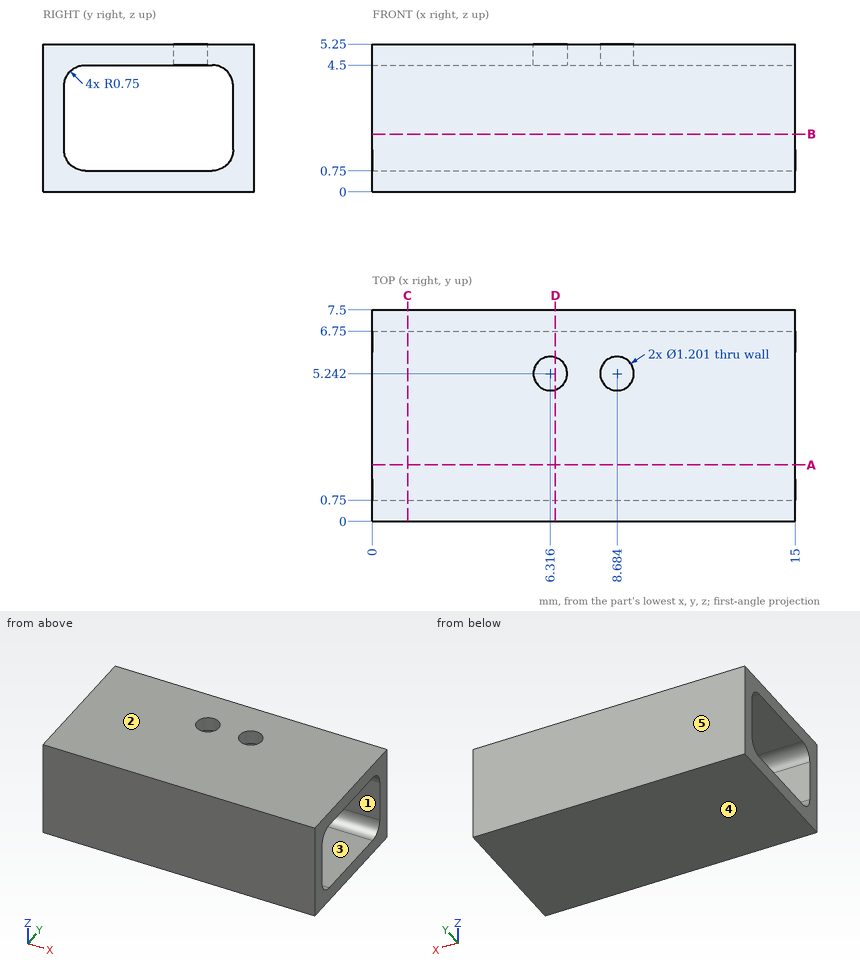
Verification items for this drawing (mm, ordinates from the low corner). A direction names the side the tool comes from. Round coordinates to 2 decimals unless told otherwise and drop trailing zeros. Loops run counter-clockwise (first coordinate to the right, second up) from the corner with the lowest first, then second, coordinate; pieces in that order, holes last. Notation, with made-up numbers: (43.25, 66.25) - (73.25, 66.25) arc R16 cw to (73.25, 82.25) - close; hole circle Ø9 at (68, -40). An arc over 180 degrees is marked (long way). Answer as CSV lines item,"result". Start each with the question number.
Item 1: Set-up check for the marked faces 1 and 2: record each of +Z, -Z, +X, -X, +Y, -Y from which the full face is reachable in a straight line by a thin tool's end or side.
Item 2: Section check C-C (x = 1.25). Record the boundary of the cut face in (y, z).
Item 3: Depth check by flat-ended pin: P1, Ø1.1, axis at x = 6.32, y = 5.24, coming from the +Z side. Enter the tip coordinate at first touch or a pass-through.
Item 4: Section check A-A (y = 2). Record the boundary of the cut face in (x, z), and give its area (3 significant figures).
Item 5: Scan lines: line 1 (Z direction, x = 14, y = 6); line 2 (Y direction, x = 13.25, z = 1.7). Record each from-to range of solid material in increasing order. Write a range as [from, to].
Item 6: Release check for a two-part mould opening along Y. For the marked faces 3, 4 and 5 record: +Y half, -Y half, draft (parallel to the pull), parting line (faces both ways), or undercut.
Item 7: Section check D-D (x = 6.5). Record the boundary of the cut face in (y, z).
Item 8: Section check B-B (z = 2.05). Record the boundary of the cut face in (x, y), and give its area (3 significant figures).
Report:
1,face 1,"+X, -X"
1,face 2,"+Z, +X, -X, +Y, -Y"
2,outline,"(0, 0) - (7.5, 0) - (7.5, 5.25) - (0, 5.25) - close; hole (0.75, 1.5) arc R0.75 ccw to (1.5, 0.75) - (6, 0.75) arc R0.75 ccw to (6.75, 1.5) - (6.75, 3.75) arc R0.75 ccw to (6, 4.5) - (1.5, 4.5) arc R0.75 ccw to (0.75, 3.75) - close"
3,P1,"stops at z = 0.75"
4,outline,"(0, 0) - (15, 0) - (15, 0.75) - (0, 0.75) - close; (0, 4.5) - (15, 4.5) - (15, 5.25) - (0, 5.25) - close"
4,area,"22.5 mm2"
5,line 1,"z = [0, 0.75], [4.5, 5.25]"
5,line 2,"y = [0, 0.75], [6.75, 7.5]"
6,face 3,"undercut"
6,face 4,"draft"
6,face 5,"+Y half"
7,outline,"(0, 0) - (7.5, 0) - (7.5, 5.25) - (5.81, 5.25) - (5.81, 4.5) - (6, 4.5) arc R0.75 cw to (6.75, 3.75) - (6.75, 1.5) arc R0.75 cw to (6, 0.75) - (1.5, 0.75) arc R0.75 cw to (0.75, 1.5) - (0.75, 3.75) arc R0.75 cw to (1.5, 4.5) - (4.67, 4.5) - (4.67, 5.25) - (0, 5.25) - close"
8,outline,"(0, 0) - (15, 0) - (15, 0.75) - (0, 0.75) - close; (0, 6.75) - (15, 6.75) - (15, 7.5) - (0, 7.5) - close"
8,area,"22.5 mm2"
